from build123d import *

# Parameters (mm, degrees)
SKETCH_1_R          = 5
SKETCH_1_R_2        = 4.505
SKETCH_1_R_3        = 1.3
SKETCH_1_R_4        = 1.5
SKETCH_1_W          = 5
SKETCH_1_H          = 10
EXTRUDE_1_DEPTH     = 4
SKETCH_2_R          = 6.01
CUT_EXTRUDE_1_DEPTH = 1
CUT_EXTRUDE_4_DEPTH = 4
FILLET_1_R          = 10


with BuildPart() as part:
    # 草图1 → 凸台-拉伸1 (new body)
    with BuildSketch(Plane(origin=(0, 0, 0), x_dir=(1, 0, 0), z_dir=(0, 1, 0))):
        with BuildLine():
            Line((150, 13), (21.354156504, 13))
            ThreePointArc((21.354156504, 13), (17.988228463, 17.361556288), (13.748715927, 20.879961934))
            Line((13.748715927, 20.879961934), (-13.748715927, 20.879961934))
            ThreePointArc((-13.748715927, 20.879961934), (-17.67766953, 17.67766953), (-20.879961934, 13.748715927))
            Line((-20.879961934, 13.748715927), (-20.879961934, -13.748715927))
            ThreePointArc((-20.879961934, -13.748715927), (-17.67766953, -17.67766953), (-13.748715927, -20.879961934))
            Line((-13.748715927, -20.879961934), (13.748715927, -20.879961934))
            ThreePointArc((13.748715927, -20.879961934), (17.988228463, -17.361556288), (21.354156504, -13))
            Line((21.354156504, -13), (150, -13))
            ThreePointArc((150, -13), (163, 0), (150, 13))
        make_face()
        with Locations(Location((0, 0, 0), (0, 0, 270))):
            Circle(SKETCH_1_R, mode=Mode.SUBTRACT)
        with Locations(Location((150, 0, 0), (0, 0, 270))):
            Circle(SKETCH_1_R_2, mode=Mode.SUBTRACT)
        with Locations(Location((120.4195, 0, 0), (0, 0, 270))):
            Circle(SKETCH_1_R_2, mode=Mode.SUBTRACT)
        with Locations(Location((0, 9, 0), (0, 0, 270))):
            Circle(SKETCH_1_R_3, mode=Mode.SUBTRACT)
        with Locations(Location((7.794228634, -4.5, 0), (0, 0, 270))):
            Circle(SKETCH_1_R_3, mode=Mode.SUBTRACT)
        with Locations(Location((-7.794228634, -4.5, 0), (0, 0, 270))):
            Circle(SKETCH_1_R_3, mode=Mode.SUBTRACT)
        with Locations(Location((135, 0, 0), (0, 0, 270))):
            Circle(SKETCH_1_R_4, mode=Mode.SUBTRACT)
        with Locations(Location((62, 0, 0), (0, 0, 270))):
            Circle(SKETCH_1_R_4, mode=Mode.SUBTRACT)
        with Locations(Location((62, 9, 0), (0, 0, 270))):
            Circle(SKETCH_1_R_4, mode=Mode.SUBTRACT)
        with Locations(Location((62, -9, 0), (0, 0, 270))):
            Circle(SKETCH_1_R_4, mode=Mode.SUBTRACT)
        with Locations(Location((-15.556349186, 15.556349186, 0), (0, 0, 270))):
            Circle(SKETCH_1_R_4, mode=Mode.SUBTRACT)
        with Locations(Location((15.556349186, 15.556349186, 0), (0, 0, 270))):
            Circle(SKETCH_1_R_4, mode=Mode.SUBTRACT)
        with Locations(Location((15.556349186, -15.556349186, 0), (0, 0, 270))):
            Circle(SKETCH_1_R_4, mode=Mode.SUBTRACT)
        with Locations(Location((-15.556349186, -15.556349186, 0), (0, 0, 270))):
            Circle(SKETCH_1_R_4, mode=Mode.SUBTRACT)
        with Locations((0, -11.773380776)):
            Rectangle(SKETCH_1_W, SKETCH_1_H, mode=Mode.SUBTRACT)
        with BuildLine():
            Line((49.912097798, -6), (19.912097798, -6))
            ThreePointArc((19.912097798, -6), (13.912097798, 0), (19.912097798, 6))
            Line((19.912097798, 6), (49.912097798, 6))
            ThreePointArc((49.912097798, 6), (55.912097798, 0), (49.912097798, -6))
        make_face(mode=Mode.SUBTRACT)
        with BuildLine():
            Line((105.041482469, -6), (75.041482469, -6))
            ThreePointArc((75.041482469, -6), (69.041482469, 0), (75.041482469, 6))
            Line((75.041482469, 6), (105.041482469, 6))
            ThreePointArc((105.041482469, 6), (111.041482469, 0), (105.041482469, -6))
        make_face(mode=Mode.SUBTRACT)
    extrude(amount=EXTRUDE_1_DEPTH)

    # 草图2 → 切除-拉伸1 (cut)
    with BuildSketch(Plane.XZ):
        with Locations(Location((150, 0, 0), (0, 0, 270))):
            Circle(SKETCH_2_R)
        with Locations(Location((120.4195, 0, 0), (0, 0, 270))):
            Circle(SKETCH_2_R)
    extrude(amount=-CUT_EXTRUDE_1_DEPTH, mode=Mode.SUBTRACT)

    # 草图4 → 切除-拉伸4 (cut)
    with BuildSketch(Plane(origin=(0, 4, 0), x_dir=(1, 0, 0), z_dir=(0, 1, 0))):
        with BuildLine():
            Line((127.5, 11), (142.5, 11))
            ThreePointArc((142.5, 11), (144.5, 9), (142.5, 7))
            Line((142.5, 7), (127.5, 7))
            ThreePointArc((127.5, 7), (125.5, 9), (127.5, 11))
        make_face()
        with BuildLine():
            Line((127.5, -11), (142.5, -11))
            ThreePointArc((142.5, -11), (144.5, -9), (142.5, -7))
            Line((142.5, -7), (127.5, -7))
            ThreePointArc((127.5, -7), (125.5, -9), (127.5, -11))
        make_face()
    extrude(amount=-CUT_EXTRUDE_4_DEPTH, mode=Mode.SUBTRACT)

    # 圆角1
    fillet_1_edges = [part.edges().sort_by_distance(p)[0] for p in [
        (21.354156504, 2, 13),
        (13.748715927, 2, 20.879961934),
        (-13.748715927, 2, 20.879961934),
        (-20.879961934, 2, 13.748715927),
        (-20.879961934, 2, -13.748715927),
        (-13.748715927, 2, -20.879961934),
        (13.748715927, 2, -20.879961934),
        (21.354156504, 2, -13),
    ]]
    fillet(fillet_1_edges, radius=FILLET_1_R)


solid = part.part
Geometry: final body of the model. Coordinates: model frame, mm. A direction names the side the tool comes from. Give positions to 0.01 mm unless a question says otherwise; leave off trailing zeros. Loops run counter-clockwise (first coordinate to the right, second up) from the corner with the lowest first, then second, coordinate; pieces in that order, holes last. Notation, with made-up numbers: (24.25, 42) -> (44.25, 42) arc R8 cw to (44.25, 57) -> close; hole circle Ø2 at (-24, 55.25). An arc over 180 degrees is marked (long way). Put each result on its own line as item: value.
1. Cut plane A-A (x = 72). Return the cut outline in (y, z).
Taken from the geometry:
outline: (0, -13) -> (4, -13) -> (4, -5.17) -> (0, -5.17) -> close; (0, 5.17) -> (4, 5.17) -> (4, 13) -> (0, 13) -> close
2. Cut plane B-B (y = 3.15). Count the separate pieces of the cut face and the enclosed holes in it, plus the area to 3 significant figures.
Taken from the geometry:
separate pieces: 1
enclosed holes: 19
area: 3,860 mm2
3. Pin query (flat end, axial travel): P1, Ø7, axis at x = 120.42, z = 0, coming from the +Y side; P2, Ø1, axis at x = 126, y = 3.5, coming from the +Z side; P3, Ø1.2, axis at y = 2.5, z = 13.5, coming from the -X side; P4, Ø6, axis at x = 122.5, z = -1.5, coming from the -Y side. Return the tip coordinate at first contact, or that it passes through.
Taken from the geometry:
P1: passes through
P2: stops at z = 13
P3: stops at x = -20.54
P4: stops at y = 1
4. Ray query, line 1 along Z through (x, y) = (15, 3.2); line 2 along X through (y, z) = (2.1, -15.5); line 3 along Z through (x, y) = (130, 2). Return the intervals inside material, ascending. Write a range as [from, to].
Taken from the geometry:
line 1: z = [-19.72, -16.95], [-14.16, -3.45], [3.45, 14.16], [16.95, 19.72]
line 2: x = [-19.44, -17.06], [-14.06, 14.06], [17.06, 19.77]
line 3: z = [-13, -11], [-7, 7], [11, 13]
5. Set-up query: faces 1 (the flat face through (116, 1, 2)), 2 (the cylindrical face through (-20.15, 2.03, -14.08)), 3 (the flat face through (90, 2, 6)). Return all of +Z, -Z, +X, -X, +Y, -Y with unobstructed straight access to the full face (end or side cutting, diameter ignored); none if empty.
Taken from the geometry:
face 1: -Y
face 2: -Z, -X, +Y, -Y
face 3: +Y, -Y
6. Pull-direction query (Z, two-part tool) for faces 4 (the cylindrical face through (155.96, 0.49, 0.78)), 5 (the flat face through (49, 0, -10)), 6 (the flat face through (89, 2, -13)); classes: released by +Z, released by -Z, zero draft, split by the parting line, or undercut.
Taken from the geometry:
face 4: undercut
face 5: zero draft
face 6: released by -Z
